Design review of the part built by this model. Coordinates are the model's own, in mm. A direction names the side the tool comes from. Give positions to 0.01 mm unless a question says otherwise; leave off trailing zeros. Answer as a JSON object with one key per item and string values.
from build123d import *

# Parameters (mm, degrees)
EXTRUDE_1_DEPTH     = 5
CUT_EXTRUDE_START   = -1
CUT_EXTRUDE_3_DEPTH = 1


# Read off the part's stored shape, not the designer's step: Вырез-Вытянуть3
with BuildPart() as part:
    # Эскиз1 → Бобышка-Вытянуть1 (new body)
    with BuildSketch(Plane.XY):
        with BuildLine():
            Line((5, 0), (57, 0))
            ThreePointArc((57, 0), (60.535533906, 1.464466094), (62, 5))
            Line((62, 5), (62, 83))
            ThreePointArc((62, 83), (60.535533906, 86.535533906), (57, 88))
            Line((57, 88), (5, 88))
            ThreePointArc((5, 88), (1.464466094, 86.535533906), (0, 83))
            Line((0, 83), (0, 5))
            ThreePointArc((0, 5), (1.464466094, 1.464466094), (5, 0))
        make_face()
    extrude(amount=EXTRUDE_1_DEPTH)

    # Вырез-Вытянуть3 outline → Вырез-Вытянуть3 (cut)
    with BuildSketch(Plane.XY.offset(5).offset(CUT_EXTRUDE_START)):
        with BuildLine():
            add(Edge.make_bspline(
                [(7.322115385, 77.948717949), (7.280403728, 77.949629189), (7.199154126, 77.951404182), (7.08103096, 77.965514138), (6.970032623, 77.986734715), (6.86753928, 78.020868189), (6.771471542, 78.06080497), (6.683688955, 78.112132534), (6.602688938, 78.171353702), (6.530522286, 78.24100741), (6.465447665, 78.318830964), (6.41163812, 78.407249412), (6.364084469, 78.503063707), (6.328183734, 78.608942585), (6.298735587, 78.722922407), (6.2805208, 78.846457423), (6.268556671, 78.978392008), (6.269001965, 79.069415592), (6.269230769, 79.116185897)],
                knots=[0, 0, 0, 0, 0.069384338, 0.135152862, 0.197735709, 0.257048427, 0.31458961, 0.370543528, 0.425833354, 0.481158895, 0.537040397, 0.594138756, 0.652974992, 0.714682156, 0.779789612, 0.848620873, 0.922217432, 1, 1, 1, 1], degree=3))
            add(Edge.make_bspline(
                [(8.423076923, 79.28525641), (8.422846482, 79.24465196), (8.422400519, 79.16607163), (8.416777036, 79.051655992), (8.406996568, 78.94425203), (8.394710578, 78.843624109), (8.377857705, 78.749984901), (8.357009271, 78.663646779), (8.333382771, 78.583908695), (8.296299771, 78.48874028), (8.239839042, 78.380770097), (8.153444079, 78.266259522), (8.049022592, 78.168573661), (7.9277584, 78.088174586), (7.79256156, 78.026127128), (7.645762848, 77.981077752), (7.487701683, 77.953199535), (7.378323021, 77.950239206), (7.322115385, 77.948717949)],
                knots=[0, 0, 0, 0, 0.061211027, 0.118459496, 0.172633106, 0.223776859, 0.271245742, 0.315976481, 0.35763086, 0.396515037, 0.469825178, 0.540534635, 0.611753614, 0.684345849, 0.758929938, 0.835221686, 0.915323526, 1, 1, 1, 1], degree=3))
            Line((8.423076923, 79.28525641), (8.423076923, 82))
            Line((8.423076923, 82), (7.858974359, 82))
            Line((7.858974359, 82), (7.858974359, 79.249198718))
            add(Edge.make_bspline(
                [(7.345352564, 78.41025641), (7.372975773, 78.411180822), (7.4269515, 78.412987123), (7.504373326, 78.431551652), (7.576511792, 78.459404941), (7.641326576, 78.500074876), (7.699113429, 78.549562242), (7.748268345, 78.607960428), (7.785711282, 78.675450105), (7.809293621, 78.737761499), (7.823759213, 78.793221645), (7.83322618, 78.841401042), (7.841207325, 78.895150355), (7.847235632, 78.954806458), (7.853355796, 79.020196267), (7.855800765, 79.091605618), (7.858650581, 79.16851443), (7.858863947, 79.221684424), (7.858974359, 79.249198718)],
                knots=[0, 0, 0, 0, 0.073594239, 0.143803085, 0.211314618, 0.27917152, 0.346904743, 0.413716382, 0.481711687, 0.551880712, 0.590958341, 0.634577158, 0.682868024, 0.735927242, 0.794594596, 0.858103432, 0.926571669, 1, 1, 1, 1], degree=3))
            add(Edge.make_bspline(
                [(6.833333333, 79.179487179), (6.834857441, 79.143941678), (6.83777302, 79.075944064), (6.84743928, 78.978324165), (6.860933127, 78.889536466), (6.877643129, 78.809256715), (6.897109916, 78.737429188), (6.921534218, 78.674633381), (6.947839007, 78.619549931), (6.980181111, 78.573892339), (7.014857408, 78.53487098), (7.053004363, 78.501738163), (7.094129871, 78.473504515), (7.138151962, 78.450181335), (7.185565934, 78.432291412), (7.235878922, 78.419864447), (7.289505669, 78.411261561), (7.326352813, 78.410598374), (7.345352564, 78.41025641)],
                knots=[0, 0, 0, 0, 0.102038713, 0.195197389, 0.281231404, 0.35951733, 0.430343554, 0.494370791, 0.552618194, 0.604901828, 0.654275293, 0.702059837, 0.749449665, 0.797086574, 0.844612455, 0.894412072, 0.945554958, 1, 1, 1, 1], degree=3))
            Line((6.833333333, 79.179487179), (6.269230769, 79.116185897))
        make_face()
        with BuildLine():
            ThreePointArc((10.5, 73.3), (8.885670907, 74.522967675), (7.5, 76))
            ThreePointArc((7.5, 76), (6.114329093, 74.522967675), (4.5, 73.3))
            ThreePointArc((4.5, 73.3), (3.605830756, 72.578400365), (2.9, 71.67173195))
            ThreePointArc((2.9, 71.67173195), (2.944094794, 68.407366911), (6.1, 67.57173195))
            Line((6.1, 67.57173195), (7.2, 68.17173195))
            ThreePointArc((7.2, 68.17173195), (6.807193425, 66.949612307), (5.7, 66.3))
            Line((5.7, 66.3), (5, 66.3))
            Line((5, 66.3), (5, 66))
            Line((5, 66), (10, 66))
            Line((10, 66), (10, 66.3))
            Line((10, 66.3), (9.3, 66.3))
            ThreePointArc((9.3, 66.3), (8.192806575, 66.949612307), (7.8, 68.17173195))
            Line((7.8, 68.17173195), (8.9, 67.57173195))
            ThreePointArc((8.9, 67.57173195), (12.055905206, 68.407366911), (12.1, 71.67173195))
            ThreePointArc((12.1, 71.67173195), (11.394169244, 72.578400365), (10.5, 73.3))
        make_face()
    extrude(amount=CUT_EXTRUDE_3_DEPTH, mode=Mode.SUBTRACT)


solid = part.part
(1) Draft analysis for pull direction Y (two halves, no side actions). For faces 3 (the cylindrical face through (12.025, 68.369, 4.493)), 4 (the cylindrical face through (61, 86, 2)), 5 (the flat face through (0, 45, 2)), state which applies: +Y half, -Y half, draft (parallel to the pull), parting line (faces both ways), or undercut.
Checked values:
{"face 3": "undercut", "face 4": "+Y half", "face 5": "draft"}
(2) Tool access review of faces 1 (the flat face through (8.1, 79.5, 4)), 2 (the flat face through (31, 45, 5)): name each direction out of +Z, -Z, +X, -X, +Y, -Y from which nothing blocks a thin tool from reaching the whole face with its end or side.
Checked values:
{"face 1": "+Z", "face 2": "+Z, +X, -X, +Y, -Y"}
(3) To check wall thickness, follow L1, parallel to X at y = 75, z = 4.65; L2, parallel to X at y = 71.5, z = 4.05; L3, parallel to Y at x = 11, z = 4.55. State the ranges of each line that lie inside material, in increasing order. Write a range as from..to.
Checked values:
{"L1": "x = 0..6.61, 8.39..62", "L2": "x = 0..2.78, 12.22..62", "L3": "y = 0..67.59, 72.94..88"}
